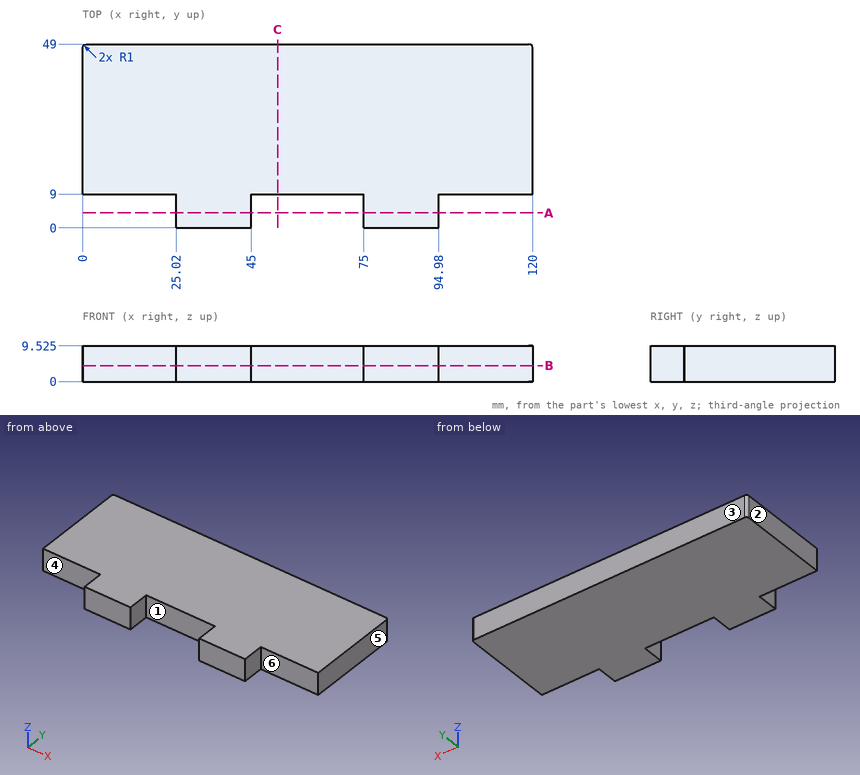
Could you check a few things on this drawing? It's one solid part, dimensions in mm from its lowest x, y, z. A direction names the side the tool comes from. Coordinates: 2 decimals unless noted, no trailing zeros. Write each loop counter-clockwise with the first axis right and the second up, starting at its lowest first coordinate (ties: lowest second). Pieces come first, ordered by that corner, then holes. Notation, with made-up numbers: (77, -34) - (109, -34) arc R22 ccw to (109, -6) - close; hole circle Ø8 at (0.5, 80.5). An arc over 180 degrees is marked (long way). Return JSON: item names as keys, results as strings. Group by question number.
Item 1: I'm going to push flat-ended pins straight in: pin 1 Ø2.5 at (y, z) = (5.5, 5.5) entering from -X; pin 2 Ø3 at (x, z) = (17.5, 6) entering from -Y; pin 3 Ø2.5 at (y, z) = (6.5, 6) entering from +X. Where does each tip first touch, or does it pass through?
Item 2: If we section it at A-A (y = 4): Write out the boundary of the cut face in (x, z) (3 decimals).
Item 3: Please list where this line runs through material, in increasing order: probe 1 along Y at (x, z) = (54, 5.25).
Item 4: If we section it at B-B (z = 4.25): Write out the boundary of the cut face in (x, y), then the cut area to 3 significant figures.
Item 5: Which directions (+Z, -Z, +X, -X, +Y, -Y) give clear straight access to the entire face, cutting with the end or side of a thin tool? Please do the marked faces 4, 5 and 6.
Item 6: If we section it at C-C (x = 52): Write out the boundary of the cut face in (y, z) (3 decimals).
Item 7: We'd pull the mould along X, two halves only. Please class the marked faces 1, 2 and 3: pulls with the +X half, pulls with the -X half, needs draft (parallel to the pull), parting line crosses it, or undercut.
Return value:
{
 "1": {"pin 1": "stops at x = 25.02", "pin 2": "stops at y = 9", "pin 3": "stops at x = 94.98"},
 "2": {"outline": "(25.02, 0) - (45, 0) - (45, 9.525) - (25.02, 9.525) - close; (75, 0) - (94.98, 0) - (94.98, 9.525) - (75, 9.525) - close"},
 "3": {"probe 1": "y = 9 to 49"},
 "4": {"outline": "(0, 9) - (25.02, 9) - (25.02, 0) - (45, 0) - (45, 9) - (75, 9) - (75, 0) - (94.98, 0) - (94.98, 9) - (120, 9) - (120, 48) arc R1 ccw to (119, 49) - (1, 49) arc R1 ccw to (0, 48) - close", "area": "5,160 mm^2"},
 "5": {"face 4": "+Z, -Z, -X, -Y", "face 5": "+Z, -Z, +X, +Y, -Y", "face 6": "+Z, -Z, +X, -Y"},
 "6": {"outline": "(9, 0) - (49, 0) - (49, 9.525) - (9, 9.525) - close"},
 "7": {"face 1": "undercut", "face 2": "pulls with the -X half", "face 3": "needs draft"}
}
